```python
from build123d import *

# Parameters (mm, degrees)
SKETCH_1_W          = 200
SKETCH_1_H          = 200
EXTRUDE_1_DEPTH     = 12
SKETCH_3_W          = 320
SKETCH_3_H          = 20
EXTRUDE_3_DEPTH     = 100
CUT_EXTRUDE_4_DEPTH = 304.716973513


with BuildPart() as part:
    # 草图1 → 拉伸1 (new body)
    with BuildSketch(Plane.XY):
        with Locations((100, 100)):
            Rectangle(SKETCH_1_W, SKETCH_1_H)
    extrude(amount=EXTRUDE_1_DEPTH)

    # 草图3 → 拉伸3 (add)
    with BuildSketch(Plane.XY.offset(12)):
        with Locations((100, 100)):
            Rectangle(SKETCH_3_W, SKETCH_3_H)
    extrude(amount=EXTRUDE_3_DEPTH)

    # 草图4 → 拉伸4 (cut, through all)
    with BuildSketch(Plane.XZ.offset(-90)):
        Polygon((200, 12), (260, 42), (260, 12), align=None)
        Polygon((-60, 42), (0, 12), (-60, 12), align=None)
    extrude(amount=-CUT_EXTRUDE_4_DEPTH, mode=Mode.SUBTRACT)


solid = part.part
```
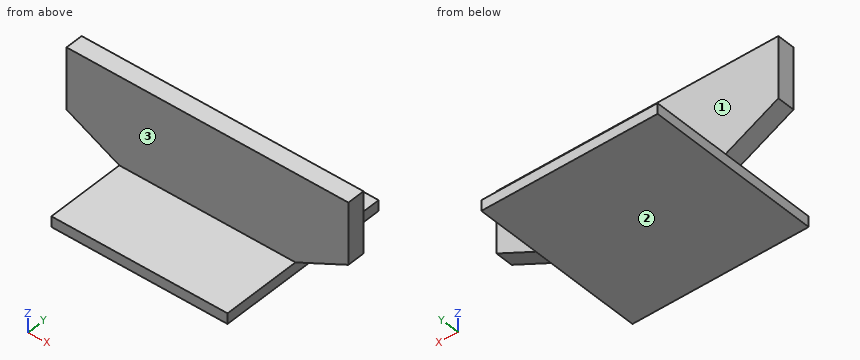
The model under review builds one solid part; all positions refer to its coordinate system, in mm. Face numbers are marked on the shaded views. A direction names the side the tool comes from. Round coordinates to 2 decimals unless told otherwise and drop trailing zeros. Order: outer loops, then holes, each group sorted by start corner. A loop starts at its lowest first (then second) coordinate and runs counter-clockwise, first axis right, second up. Notation, with made-up numbers: (67.25, 8) -> (123.25, 8) arc R7 ccw to (123.25, 18) -> close; hole circle Ø1 at (-24, 78). An arc over 180 degrees is marked (long way). Use a Markdown table: item, result.
Q1. We need section C-C on z = 21.5. Write out the cut boundary in (x, y), then the cut area to 3 significant figures.
Values:
| item | result |
|---|---|
| outline | (-19, 90) -> (219, 90) -> (219, 110) -> (-19, 110) -> close |
| area | 4,760 mm^2 |
Q2. We need section A-A on x = 34.5. Write out the cut boundary in (y, z).
Values:
| item | result |
|---|---|
| outline | (0, 0) -> (200, 0) -> (200, 12) -> (110, 12) -> (110, 112) -> (90, 112) -> (90, 12) -> (0, 12) -> close |
Q3. For line 1 (Z direction, x = 3.5, y = 68); line 2 (Y direction, x = 231.5, z = 104.5); line 3 (X direction, y = 61, z = 11), list the stretches that pass through material, from the lowest coordinate up.
Values:
| item | result |
|---|---|
| line 1 | z = 0 to 12 |
| line 2 | y = 90 to 110 |
| line 3 | x = 0 to 200 |
Q4. We need section B-B on y = 67. Write out the cut boundary in (x, z).
Values:
| item | result |
|---|---|
| outline | (0, 0) -> (200, 0) -> (200, 12) -> (0, 12) -> close |
Q5. Clearance check with flat-ended pins moving along their axes: P1, Ø1.5, axis at x = 108, z = 70, coming from the +Y side; P2, Ø13, axis at y = 140.5, z = 5.5, coming from the +X side; P3, Ø5, axis at y = 101, z = 34.5, coming from the -X side. State where each tip first meets the part, or that it passes through.
Values:
| item | result |
|---|---|
| P1 | stops at y = 110 |
| P2 | stops at x = 200 |
| P3 | stops at x = -50 |
Q6. Tool access review of the marked faces 1, 2 and 3: name each direction out of +Z, -Z, +X, -X, +Y, -Y from which nothing blocks a thin tool from reaching the whole face with its end or side.
Values:
| item | result |
|---|---|
| face 1 | +Z, +X, -X, +Y |
| face 2 | -Z, +X, -X, +Y, -Y |
| face 3 | +Z, +X, -X, -Y |
